For this review, use the dimensioned drawing (mm, ordinates from the lowest corner) and the shaded views. Coordinates: 2 decimals unless noted, no trailing zeros. Loops run counter-clockwise (first coordinate to the right, second up) from the corner with the lowest first, then second, coordinate; pieces in that order, holes last.
1. Take a section at B-B, the plane z = 1.65. State the section outline as (x, y) points.
2. Take a section at A-A, the plane x = 5. State the section outline as (y, z) points, then the cut area to 3 significant figures.
3. Take a section at C-C, the plane y = 3.15. State the section outline as (x, z) points, then the cut area to 3 significant figures.
4. Take a section at D-D, the plane x = 24.5. State the section outline as (y, z) points.
5. To check wall thickness, follow probe 1 along X at (y, z) = (2.75, 0.95); probe 2 along Y at (x, z) = (5, 0.65); probe 3 along Y at (x, z) = (6, 0.5). State the ranges of each line that lie inside material, in increasing order.
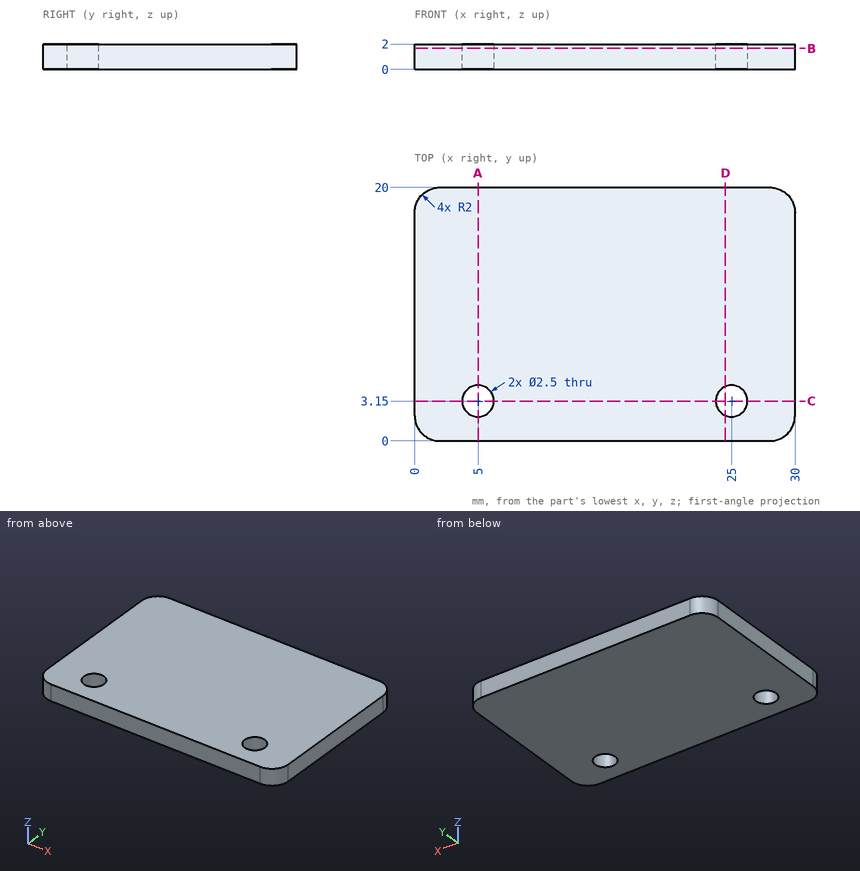
Results list:
1. outline: (0, 2) arc R2 ccw to (2, 0) - (28, 0) arc R2 ccw to (30, 2) - (30, 18) arc R2 ccw to (28, 20) - (2, 20) arc R2 ccw to (0, 18) - close; hole circle Ø2.5 at (5, 3.15); hole circle Ø2.5 at (25, 3.15)
2. outline: (0, 0) - (1.9, 0) - (1.9, 2) - (0, 2) - close; (4.4, 0) - (20, 0) - (20, 2) - (4.4, 2) - close
2. area: 35.0 mm2
3. outline: (0, 0) - (3.75, 0) - (3.75, 2) - (0, 2) - close; (6.25, 0) - (23.75, 0) - (23.75, 2) - (6.25, 2) - close; (26.25, 0) - (30, 0) - (30, 2) - (26.25, 2) - close
3. area: 50.0 mm2
4. outline: (0, 0) - (2, 0) - (2, 2) - (0, 2) - close; (4.3, 0) - (20, 0) - (20, 2) - (4.3, 2) - close
5. probe 1: x = 0 to 3.82, 6.18 to 23.82, 26.18 to 30
5. probe 2: y = 0 to 1.9, 4.4 to 20
5. probe 3: y = 0 to 2.4, 3.9 to 20
